from build123d import *

# Parameters (mm, degrees)
F0_R     = 3.175
F1_DEPTH = 2.54
F2_R     = 12.7


with BuildPart() as f1:
    # F0 (on Top) → F1 (new body)
    with BuildSketch(Plane.XY):
        Polygon((-318.52108, 0), (0, 0), (-255.939342, 300.836124), align=None)
        with Locations((-295.100357, 19.05)):
            Circle(F0_R, mode=Mode.SUBTRACT)
        with Locations((-169.663504, 19.05)):
            Circle(F0_R, mode=Mode.SUBTRACT)
        with Locations((-270.480821, 137.398359)):
            Circle(F0_R, mode=Mode.SUBTRACT)
        with Locations((-223.245375, 75.209031)):
            Circle(F0_R, mode=Mode.SUBTRACT)
        with Locations((-41.218348, 19.05)):
            Circle(F0_R, mode=Mode.SUBTRACT)
        with Locations((-143.615105, 75.209031)):
            Circle(F0_R, mode=Mode.SUBTRACT)
        with Locations((-143.024825, 138.71533)):
            Circle(F0_R, mode=Mode.SUBTRACT)
        with Locations((-207.599941, 150.418062)):
            Circle(F0_R, mode=Mode.SUBTRACT)
        with Locations((-245.218643, 258.835949)):
            Circle(F0_R, mode=Mode.SUBTRACT)
    extrude(amount=F1_DEPTH)

    # F2
    f2_edges = [f1.edges().sort_by_distance(p)[0] for p in [
        (-318.52108, 0, 1.27),
        (0, 0, 1.27),
        (-255.939342, 300.836124, 1.27),
    ]]
    fillet(f2_edges, radius=F2_R)


solid = f1.part
CAD build for the part. Positions are in the model's coordinates, mm. Coordinates: 2 decimals unless noted, no trailing zeros. Order: outer loops, then holes, each group sorted by start corner. A loop starts at its lowest first (then second) coordinate and runs counter-clockwise, first axis right, second up.
Item 1: Band-saw the part on A-A on z = 0.55. Give the number of separate pieces and of enclosed holes in the cut face, plus the area to 3 significant figures.
Check sheet entries:
separate pieces: 1
enclosed holes: 9
area: 47,300 mm2
Item 2: Two-plate mould, pull along X, no slides. Class faces 1 (the face through (-242.19, 259.79, 1.25)), 2 (the face through (-16.037, 7.189, 1.288)), 3 (the face through (-201, 113, 2.54)): +X half, -X half, draft (parallel to the pull), parting line (faces both ways), or undercut.
Check sheet entries:
face 1: undercut
face 2: +X half
face 3: draft
Item 3: Drill centre lines: L1, parallel to Y at x = -210.5, z = 1.55; L2, parallel to X at y = 260, z = 0.35; L3, parallel to Y at x = -209, z = 1.25. Where is each one in solid material? Low to high.
Check sheet entries:
L1: y = 0 to 149.13, 151.71 to 247.43
L2: x = -264.43 to -248.17, -242.26 to -221.2
L3: y = 0 to 147.57, 153.27 to 245.66
Item 4: Band-saw the part on B-B on y = 227.5. List the corners of the cut face in (x, z), plus the area to 3 significant figures.
Check sheet entries:
outline: (-271.2, 0) - (-193.55, 0) - (-193.55, 2.54) - (-271.2, 2.54) - close
area: 197 mm2
Item 5: Band-saw the part on C-C on x = -75.5. List the corners of the cut face in (y, z).
Check sheet entries:
outline: (0, 0) - (88.74, 0) - (88.74, 2.54) - (0, 2.54) - close
Item 6: Pin check, flat tip, straight feed: pin 1 Ø1 at (y, z) = (127.5, 2) entering from +X. Stop position of the tip, or through.
Check sheet entries:
pin 1: stops at x = -108.05
